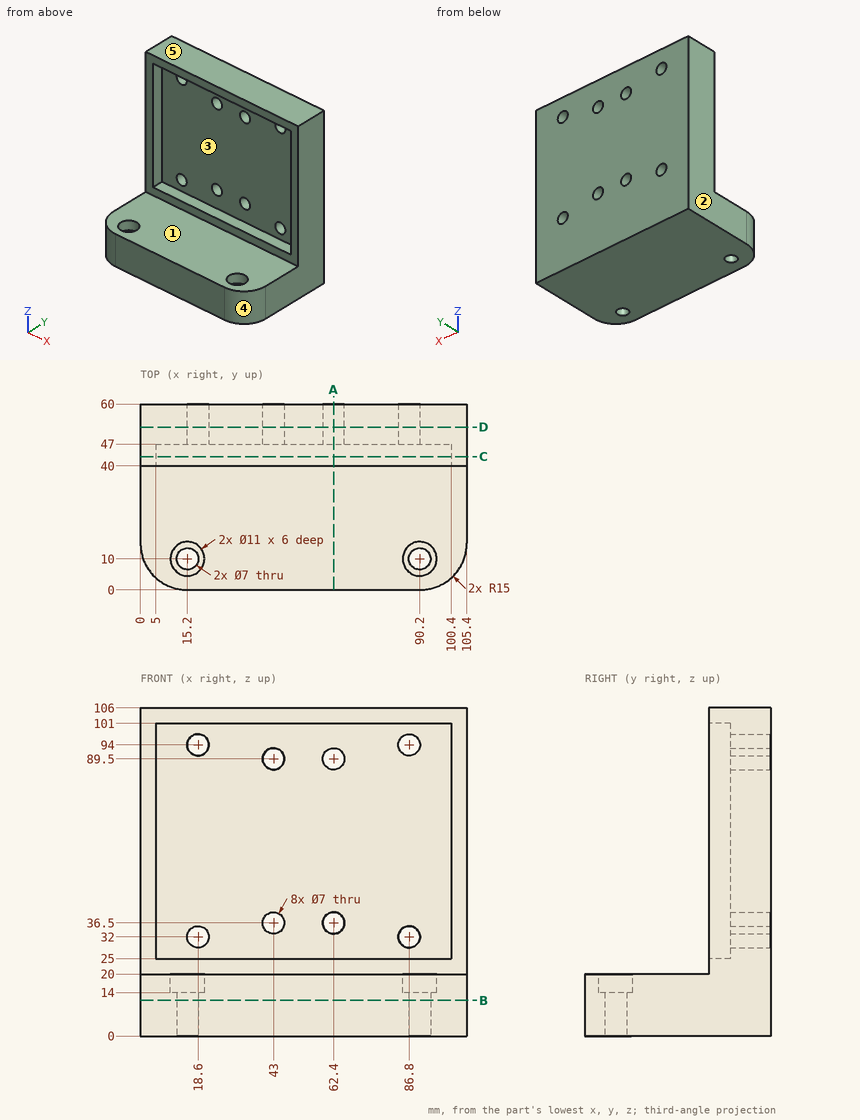
For this review, use the dimensioned drawing (mm, ordinates from the lowest corner) and the shaded views. A direction names the side the tool comes from. Coordinates: 2 decimals unless noted, no trailing zeros. Order: outer loops, then holes, each group sorted by start corner. A loop starts at its lowest first (then second) coordinate and runs counter-clockwise, first axis right, second up. Notation, with made-up numbers: (-31.75, 21.25) - (0.25, 21.25) arc R29 ccw to (0.25, 51.25) - close; hole circle Ø4 at (50, 25). An arc over 180 degrees is marked (long way). Answer in a Markdown table with one row per item.
(1) Wall thickness on line 1 along Z through (x, y) = (18.6, 51.25); line 2 along X through (y, z) = (54.25, 36.5); line 3 along Z through (x, y) = (62.4, 52): over which ranges is each line inside the solid? List them lowest first. Write a range as from..to.
Checked values:
| item | result |
|---|---|
| line 1 | 0..28.5, 35.5..90.5, 97.5..106 |
| line 2 | 0..39.5, 46.5..58.9, 65.9..105.4 |
| line 3 | 0..33, 40..86, 93..106 |
(2) Clearance check with flat-ended pins moving along their axes: pin 1 (9 mm diameter, centred on x = 15.2, y = 10, fed in from +Z); pin 2 (12.5 mm diameter, centred on x = 90.2, y = 10, fed in from +Z); pin 3 (11 mm diameter, centred on x = 18.6, z = 94, fed in from -Y). State where each tip first meets the part, or that it passes through.
Checked values:
| item | result |
|---|---|
| pin 1 | z = 14 |
| pin 2 | z = 20 |
| pin 3 | y = 47 |
(3) Consider section D-D on y = 52.5. Give the number of separate pieces and of enclosed holes in the cut face, plus the area to 3 significant figures.
Checked values:
| item | result |
|---|---|
| separate pieces | 1 |
| enclosed holes | 8 |
| area | 10,900 mm^2 |
(4) The part is to be moulded in two halves that separate along X. For the marked faces 3, 4 and 5, say which applies: released by +X, released by -X, zero draft, split by the parting line, or undercut.
Checked values:
| item | result |
|---|---|
| face 3 | undercut |
| face 4 | released by +X |
| face 5 | zero draft |
(5) For the marked faces 1 and 2, list the 3-axis set-ups (+Z, -Z, +X, -X, +Y, -Y) from which the entire face can be reached by the end or side of a thin tool; tool diameter is ignored.
Checked values:
| item | result |
|---|---|
| face 1 | +Z, +X, -X, -Y |
| face 2 | +Z, -Z, -X, +Y, -Y |
(6) Consider section C-C on y = 43. State the section outline as (x, z) points, plus the area to 3 significant figures.
Checked values:
| item | result |
|---|---|
| outline | (0, 0) - (105.4, 0) - (105.4, 106) - (0, 106) - close; hole (5, 25) - (100.4, 25) - (100.4, 101) - (5, 101) - close |
| area | 3,920 mm^2 |
(7) Consider section B-B on z = 11.5. State the section outline as (x, y) points, plus the area to 3 significant figures.
Checked values:
| item | result |
|---|---|
| outline | (0, 15) arc R15 ccw to (15, 0) - (90.4, 0) arc R15 ccw to (105.4, 15) - (105.4, 60) - (0, 60) - close; hole circle Ø7 at (15.2, 10); hole circle Ø7 at (90.2, 10) |
| area | 6,150 mm^2 |
(8) Consider section A-A on x = 62.4. State the section outline as (y, z) points.
Checked values:
| item | result |
|---|---|
| outline | (0, 0) - (60, 0) - (60, 33) - (47, 33) - (47, 25) - (40, 25) - (40, 20) - (0, 20) - close; (40, 101) - (47, 101) - (47, 93) - (60, 93) - (60, 106) - (40, 106) - close; (47, 40) - (60, 40) - (60, 86) - (47, 86) - close |
